Geometry: see drawing. Coordinates: mm, zero at the bounding-box minimum. Round coordinates to 2 decimals unless told otherwise and drop trailing zeros. Order: outer loops, then holes, each group sorted by start corner. A loop starts at its lowest first (then second) coordinate and runs counter-clockwise, first axis right, second up. Notation, with made-up numbers: (21, -11.75) -> (57, -11.75) arc R27 cw to (57, 13.25) -> close; hole circle Ø8 at (36, 21). An arc over 180 degrees is marked (long way). Answer as CSV lines item,"result". Start each with the question number.
(1) Pull-direction query (X, two-part tool) for the marked faces 1, 2 and 3; classes: +X half, -X half, draft (parallel to the pull), parting line (faces both ways), or undercut.
(2) Contact query for flat-ended pins moving along their axis: P1, Ø3, axis at y = 17.5, z = 3.5, coming from the +X side; P2, Ø2, axis at y = 5, z = 0.5, coming from the +X side. Output: stop coordinate, or through.
(3) Section query C-C (y = 10.5). Output: boundary loops of the cut face in (x, z).
(4) Section query A-A (y = 15). Output: boundary loops of the cut face in (x, z).
(5) Section query B-B (x = 15). Output: boundary loops of the cut face in (y, z).
(6) Section query D-D (z = 2.4). Output: boundary loops of the cut face in (x, y).
(7) Line query: line 1 along Y through (x, z) = (15, 4.25); line 2 along Y through (x, z) = (22.25, 4.65); line 3 along X through (y, z) = (20, 4.75) (1 decimal). Output: solid intervals per line, ascending. Write a range as from..to.
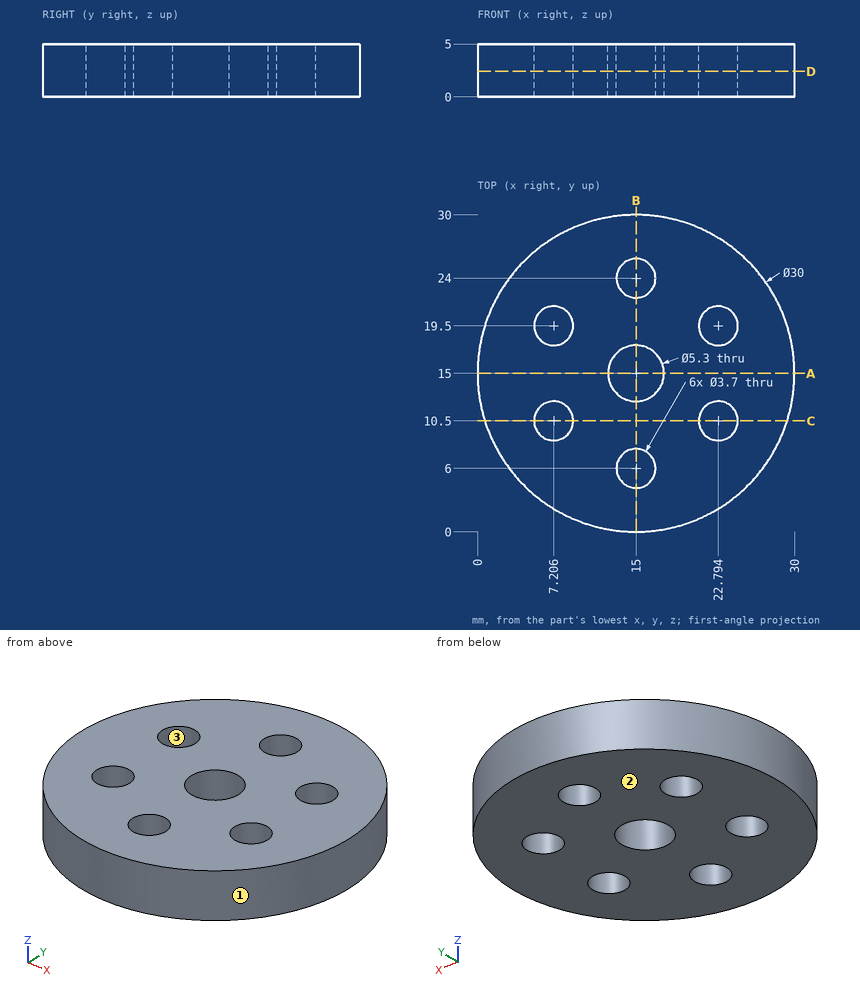
Answer block:
1,face 1,"parting line"
1,face 2,"draft"
1,face 3,"undercut"
2,P1,"x = 29.97"
2,P2,"x = 27"
3,outline,"(0.69, 0) -> (5.36, 0) -> (5.36, 5) -> (0.69, 5) -> close; (9.06, 0) -> (20.94, 0) -> (20.94, 5) -> (9.06, 5) -> close; (24.64, 0) -> (29.31, 0) -> (29.31, 5) -> (24.64, 5) -> close"
4,outline,"(0, 0) -> (12.35, 0) -> (12.35, 5) -> (0, 5) -> close; (17.65, 0) -> (30, 0) -> (30, 5) -> (17.65, 5) -> close"
5,outline,"(0, 0) -> (4.15, 0) -> (4.15, 5) -> (0, 5) -> close; (7.85, 0) -> (12.35, 0) -> (12.35, 5) -> (7.85, 5) -> close; (17.65, 0) -> (22.15, 0) -> (22.15, 5) -> (17.65, 5) -> close; (25.85, 0) -> (30, 0) -> (30, 5) -> (25.85, 5) -> close"
6,outline,"circle Ø30 at (15, 15); hole circle Ø3.7 at (7.21, 10.5); hole circle Ø3.7 at (7.21, 19.5); hole circle Ø5.3 at (15, 15); hole circle Ø3.7 at (15, 6); hole circle Ø3.7 at (15, 24); hole circle Ø3.7 at (22.79, 10.5); hole circle Ø3.7 at (22.79, 19.5)"
7,line 1,"0..4.15, 7.85..12.35, 17.65..22.15, 25.85..30"
7,line 2,"1.87..8.73, 12.27..17.73, 21.27..28.13"
7,line 3,"0.9..5.4, 9..21, 24.6..29.1"
